Verification items for this drawing (mm, ordinates from the low corner). Round coordinates to 2 decimals unless told otherwise and drop trailing zeros. Write each loop counter-clockwise with the first axis right and the second up, starting at its lowest first coordinate (ties: lowest second). Pieces come first, ordered by that corner, then holes. Notation, with made-up numbers: M -15,46.5 L 11,46.5 A16 ccw 11,53.5 Z; hole C 87.25,-2 d11. An arc over 180 degrees is marked long. One line per question, with ' | ' between items. Start each with the question number.
Q1. Gauge pin test, flat ends, axial feed: pin 1 (5.5 mm diameter, centred on x = 17.3, z = 146.17, fed in from -Y); pin 2 (10.5 mm diameter, centred on x = 93, z = 63.17, fed in from +Y). Record the tip position at first contact, or that the pin passes through.
Q2. Cross-section at B-B (y = 4.2). Record the boundary of the cut face in (x, z).
Q3. Cross-section at A-A (x = 39). Record the boundary of the cut face in (y, z).
Q4. Thickness scan on line 1 along Z through (x, y) = (38.5, 0.7) (1 decimal); line 2 along Z through (x, y) = (39, 3.2); line 3 along X through (y, z) = (4.4, 107). Record the ranges inside material, lowest first. Write a range as from..to.
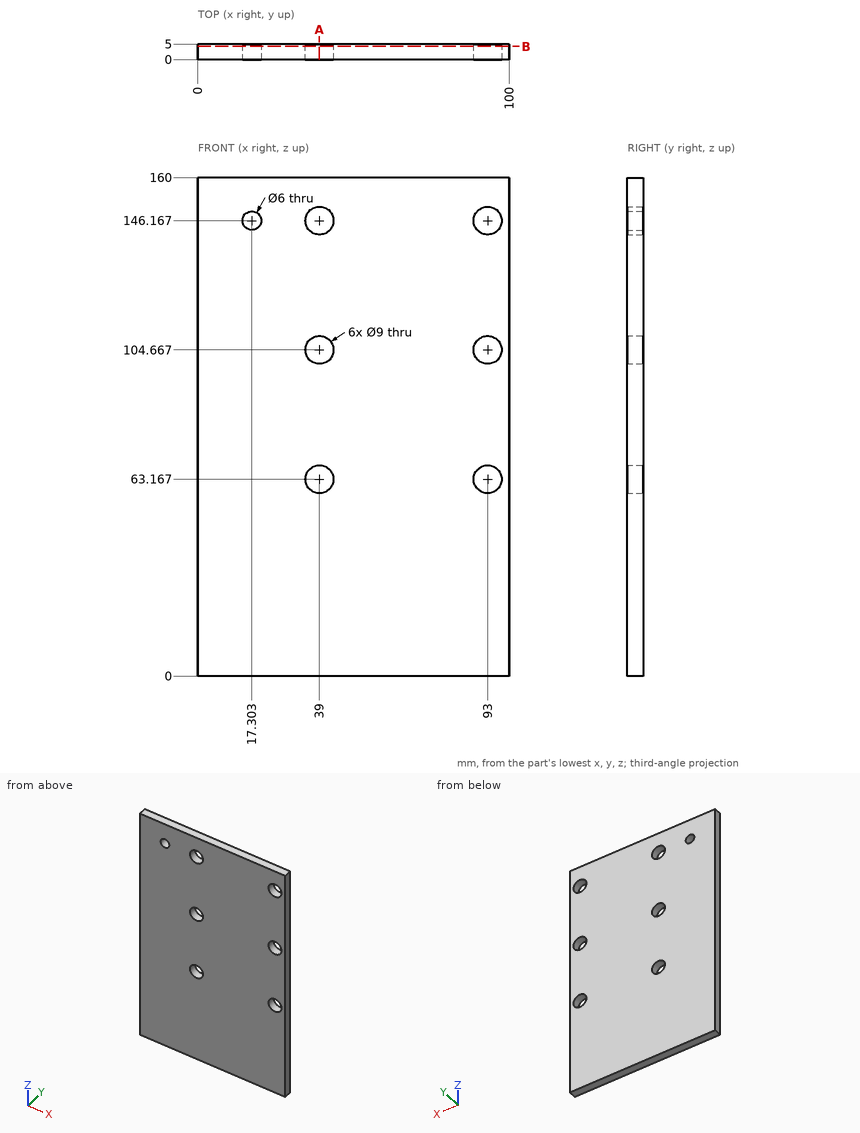
Determined:
1) pin 1: passes through | pin 2: stops at y = 5
2) outline: M 0,0 L 100,0 L 100,160 L 0,160 Z; hole C 17.3,146.17 d6; hole C 39,63.17 d9; hole C 39,104.67 d9; hole C 39,146.17 d9; hole C 93,63.17 d9; hole C 93,104.67 d9; hole C 93,146.17 d9
3) outline: M 0,0 L 5,0 L 5,58.67 L 0,58.67 Z; M 0,67.67 L 5,67.67 L 5,100.17 L 0,100.17 Z; M 0,109.17 L 5,109.17 L 5,141.67 L 0,141.67 Z; M 0,150.67 L 5,150.67 L 5,160 L 0,160 Z
4) line 1: z = 0..58.7, 67.6..100.2, 109.1..141.7, 150.6..160 | line 2: z = 0..58.67, 67.67..100.17, 109.17..141.67, 150.67..160 | line 3: x = 0..35.15, 42.85..89.15, 96.85..100
